Solid Edge part; units mm, degrees
sketch "Sketch1" plane through (0, 0, 0) normal (0, -1, 0) x (1, 0, 0)
  circle A0 centre (0, 0) radius 30
extrude "Protrusion1" add sketch "Sketch1" against normal blind 190
sketch "Sketch2" plane through (0, 0, 0) normal (0, -1, 0) x (1, 0, 0)
  circle A0 centre (0, 0) radius 45
extrude "ExtrudedProtrusion_2" add sketch "Sketch2" against normal blind 10
mirror "Mirror1" about plane through (0, 95, 0) normal (0, -1, 0) of "ExtrudedProtrusion_2"
Source: CAD feature listing. Evaluate the final solid. Frame: model axes, mm. A direction names the side the tool comes from. Coordinates: 2 decimals unless noted, no trailing zeros. Loops run counter-clockwise (first coordinate to the right, second up) from the corner with the lowest first, then second, coordinate; pieces in that order, holes last. Notation, with made-up numbers: (14, -35.75) - (19, -35.75) arc R12 ccw to (19, -30.75) - close; hole circle Ø8 at (70.25, 13.5). An arc over 180 degrees is marked (long way). Return JSON: item names as keys, results as strings.
Q1. Mould query, pull axis Y, two halves, no side actions, for faces 3 (the cylindrical face through (20.765, 185.07, 39.923)), 4 (the flat face through (-9, 180, 29)), 5 (the flat face through (1, 0, 1)). Classes: released by +Y, released by -Y, zero draft, split by the parting line, or undercut.
Results:
{"face 3": "zero draft", "face 4": "undercut", "face 5": "released by -Y"}
Q2. Section C-C, the plane z = 36.5. Return loops of the section in (x, y), plus the area to 3 significant figures.
Results:
{"outline": "(-26.32, 0) - (26.32, 0) - (26.32, 10) - (-26.32, 10) - close; (-26.32, 180) - (26.32, 180) - (26.32, 190) - (-26.32, 190) - close", "area": "1,050 mm2"}
Q3. Contact query for flat-ended pins moving along their axis: P1, Ø1.5, axis at x = 15.5, y = 147.5, coming from the -Z side; P2, Ø6, axis at y = 90.5, z = 26, coming from the +X side; P3, Ø8, axis at x = 4, y = 20.5, coming from the -Z side. Output: stop coordinate, or through.
Results:
{"P1": "z = -26.12", "P2": "x = 19.26", "P3": "z = -30"}
Q4. Material intervals for line 1 along Y through (x, z) = (21, 27.5); line 2 along X through (y, z) = (26, -18.5); line 3 along Z through (x, y) = (-20.5, 121.5), sorted ascending.
Results:
{"line 1": "0 to 10, 180 to 190", "line 2": "-23.62 to 23.62", "line 3": "-21.9 to 21.9"}
Q5. Access query for faces 1 (the cylindrical face through (20.765, 4.93, -39.923)), 2 (the cylindrical face through (-29.97, 93.81, 1.32)). Directions: +Z, -Z, +X, -X, +Y, -Y. A direction counts if a zero-diameter tool reaches every point of the face in a straight line with its end or side. Return the directions, or none.
Results:
{"face 1": "+Y, -Y", "face 2": "none"}
Q6. Section B-B, the plane z = 0. Return loops of the section in (x, y), plus the area to 3 significant figures.
Results:
{"outline": "(-45, 0) - (45, 0) - (45, 10) - (30, 10) - (30, 180) - (45, 180) - (45, 190) - (-45, 190) - (-45, 180) - (-30, 180) - (-30, 10) - (-45, 10) - close", "area": "12,000 mm2"}
Q7. Section D-D, the plane x = 0. Return loops of the section in (y, z).
Results:
{"outline": "(0, -45) - (10, -45) - (10, -30) - (180, -30) - (180, -45) - (190, -45) - (190, 45) - (180, 45) - (180, 30) - (10, 30) - (10, 45) - (0, 45) - close"}
Q8. Section A-A, the plane x = 36.5. Return loops of the section in (y, z).
Results:
{"outline": "(0, -26.32) - (10, -26.32) - (10, 26.32) - (0, 26.32) - close; (180, -26.32) - (190, -26.32) - (190, 26.32) - (180, 26.32) - close"}
